```python
from build123d import *

# Parameters (mm, degrees)
SKETCH1_W           = 25.4
SKETCH1_H           = 76.2
BOSS_EXTRUDE1_DEPTH = 50.8
SKETCH2_R           = 14.2875
CUT_EXTRUDE1_DEPTH  = 488.833224229


with BuildPart() as part:
    # Sketch1 → Boss-Extrude1 (new body)
    with BuildSketch(Plane(origin=(0, 0, 0), x_dir=(1, 0, 0), z_dir=(0, 1, 0))):
        Polygon((-279.4, 86.184650326), (-279.4, -86.184650326), (-228.6, -86.184650326), (-228.6, 35.384650326), (228.6, 35.384650326), (228.6, -86.184650326), (279.4, -86.184650326), (279.4, 86.184650326), (177.8, 86.184650326), (152.4, 86.184650326), (-152.4, 86.184650326), (-177.8, 86.184650326), align=None)
        with Locations((-165.1, 124.284650326)):
            Rectangle(SKETCH1_W, SKETCH1_H)
        with Locations((165.1, 124.284650326)):
            Rectangle(SKETCH1_W, SKETCH1_H)
    extrude(amount=BOSS_EXTRUDE1_DEPTH)

    # Sketch2 → Cut-Extrude1 (cut, through all)
    with BuildSketch(Plane(origin=(177.8, 0, 0), x_dir=(0, 0, -1), z_dir=(1, 0, 0))):
        with Locations(Location((132.85952271, 25.273316146, 0), (0, 0, 180))):
            Circle(SKETCH2_R)
    extrude(amount=-CUT_EXTRUDE1_DEPTH, mode=Mode.SUBTRACT)


solid = part.part
```
Geometry check sheet. Reference: the model listing, model coordinates, mm. A direction names the side the tool comes from. Round coordinates to 2 decimals unless told otherwise and drop trailing zeros. Write each loop counter-clockwise with the first axis right and the second up, starting at its lowest first coordinate (ties: lowest second). Pieces come first, ordered by that corner, then holes. Notation, with made-up numbers: (65, 22.5) -> (88, 22.5) arc R34 cw to (88, 56.5) -> close; hole circle Ø7 at (45, 83). An arc over 180 degrees is marked (long way). Put each result on its own line as item: value.
1) Access from +Z, -Z, +X, -X, +Y, -Y to the whole of each face (thin tool, end or side, straight path). Record for faces 5 (the face through (2, 25, -86.185)), 6 (the face through (279.4, 25, 1)), 7 (the face through (-228, 25, -86.185)), 8 (the face through (-228.6, 25, 26)), 9 (the face through (229, 25, -86.185)).
Recorded:
face 5: -Z, +Y, -Y
face 6: +Z, -Z, +X, +Y, -Y
face 7: -Z, -X, +Y, -Y
face 8: +Z, +Y, -Y
face 9: -Z, +X, +Y, -Y
2) Cross-section at C-C, the plane y = 5.5. Enter the section's corners in (x, z), plus the area to 3 significant figures.
Recorded:
outline: (-279.4, -86.18) -> (-177.8, -86.18) -> (-177.8, -162.38) -> (-152.4, -162.38) -> (-152.4, -86.18) -> (152.4, -86.18) -> (152.4, -162.38) -> (177.8, -162.38) -> (177.8, -86.18) -> (279.4, -86.18) -> (279.4, 86.18) -> (228.6, 86.18) -> (228.6, -35.38) -> (-228.6, -35.38) -> (-228.6, 86.18) -> (-279.4, 86.18) -> close
area: 44,600 mm2
3) Thickness scan on probe 1 along X at (y, z) = (11.5, -19); probe 2 along Z at (x, y) = (-88.5, 40.5); probe 3 along Z at (x, y) = (-245, 43.5). Record the ranges inside material, lowest first. Write a range as from..to.
Recorded:
probe 1: x = -279.4..-228.6, 228.6..279.4
probe 2: z = -86.18..-35.38
probe 3: z = -86.18..86.18
4) Cross-section at B-B, the plane z = -127. Enter the section's corners in (x, y).
Recorded:
outline: (-177.8, 0) -> (-152.4, 0) -> (-152.4, 12.24) -> (-177.8, 12.24) -> close; (-177.8, 38.3) -> (-152.4, 38.3) -> (-152.4, 50.8) -> (-177.8, 50.8) -> close; (152.4, 0) -> (177.8, 0) -> (177.8, 12.24) -> (152.4, 12.24) -> close; (152.4, 38.3) -> (177.8, 38.3) -> (177.8, 50.8) -> (152.4, 50.8) -> close
5) Depth check by flat-ended pin: P1, Ø3, axis at x = -117, y = 44.5, coming from the -Z side; P2, Ø15, axis at y = 21.5, z = -111.5, coming from the -X side. Enter the tip coordinate at first touch or a pass-through.
Recorded:
P1: stops at z = -86.18
P2: stops at x = -177.8
6) Release check for a two-part mould opening along X. For faces 1 (the face through (-22, 0, -39)), 2 (the face through (-177.8, 25, -115)), 3 (the face through (-3, 25, -35.385)), 4 (the face through (-152.4, 25, -115)) record: pulls with the +X half, pulls with the -X half, needs draft (parallel to the pull), parting line crosses it, or undercut.
Recorded:
face 1: needs draft
face 2: pulls with the -X half
face 3: undercut
face 4: undercut
7) Cross-section at D-D, the plane x = 170.5. Enter the section's corners in (y, z) (1 decimal).
Recorded:
outline: (0, -162.4) -> (50.8, -162.4) -> (50.8, -35.4) -> (0, -35.4) -> close; hole circle Ø28.6 at (25.3, -132.9)
8) Cross-section at A-A, the plane z = 54.5. Enter the section's corners in (x, y).
Recorded:
outline: (-279.4, 0) -> (-228.6, 0) -> (-228.6, 50.8) -> (-279.4, 50.8) -> close; (228.6, 0) -> (279.4, 0) -> (279.4, 50.8) -> (228.6, 50.8) -> close
